Read the model definition and answer for the solid it produces. Units are mm, in the model's axes. A direction names the side the tool comes from. Give positions to 0.01 mm unless a question says otherwise; leave off trailing zeros. Write each loop counter-clockwise with the first axis right and the second up, starting at its lowest first coordinate (ties: lowest second). Pieces come first, ordered by that corner, then holes. Notation, with made-up numbers: M -19,31.25 L 7,31.25 A3 ccw 7,35.25 Z; hole C 52.5,74.5 d5. An arc over 180 degrees is marked long. Write each question's results on one line, items separated by ' | '. Start each with the question number.
```python
from build123d import *

# Parameters (mm, degrees)
F0_R          = 7.9375
F1_DEPTH      = 9.525
F1_DEPTH_BACK = 50.8
F2_R          = 31.75
F3_DEPTH      = 41.275
F4_R          = 15.08125
F5_DEPTH      = 101.601
F7_DEPTH      = 76.201


with BuildPart() as f1:
    # F0 (on Top) → F1 (new body, two sides)
    with BuildSketch(Plane.XY) as f1_sk:
        with BuildLine():
            Line((-476.25, -38.1), (0, -38.1))
            ThreePointArc((0, -38.1), (38.1, 0), (0, 38.1))
            Line((0, 38.1), (-180.615451, 38.1))
            Line((-180.615451, 38.1), (-323.73747, 38.1))
            Line((-323.73747, 38.1), (-389.728606, 0))
            Line((-389.728606, 0), (-432.606556, 0))
            ThreePointArc((-432.606556, 0), (-436.495121, 1.329884), (-438.754917, 4.7625))
            ThreePointArc((-438.754917, 4.7625), (-459.600382, 18.898166), (-476.25, 0))
            Line((-476.25, 0), (-476.25, -38.1))
        make_face()
        with Locations((-457.2, 0)):
            Circle(F0_R, mode=Mode.SUBTRACT)
    extrude(amount=F1_DEPTH)
    extrude(f1_sk.sketch, amount=-F1_DEPTH_BACK)

    # F2 (on face) → F3 (join)
    with BuildSketch(Plane.XY.offset(9.525)):
        Circle(F2_R)
    extrude(amount=F3_DEPTH)

    # F4 (on face) → F5 (cut, through all)
    with BuildSketch(Plane.XY.offset(50.8)):
        Circle(F4_R)
    extrude(amount=-F5_DEPTH, mode=Mode.SUBTRACT)

    # F6 (on face) → F7 (cut, through all)
    with BuildSketch(Plane(origin=(0, 38.1, 0), x_dir=(-1, 0, 0), z_dir=(0, 1, 0))):
        Polygon((-101.6, -50.8), (254, -50.8), (166.011819, 0), (-101.6, 0), align=None)
        Polygon((524.164035, 9.525), (168.564035, 9.525), (256.552216, -41.275), (524.164035, -41.275), align=None)
    extrude(amount=-F7_DEPTH, mode=Mode.SUBTRACT)


solid = f1.part
```
Item 1: Given P1, Ø5, axis at x = -421, z = -48, coming from the +Y side; P2, Ø1.5, axis at y = -16, z = 22.5, coming from the -X side; P3, Ø4, axis at x = -16.5, y = -19, coming from the -Z side, each flat-ended and moving along its own axis, determine where each tip first touches the part or whether it passes through.
Item 2: Section C-C, the plane x = -161 is taken. Determine the outline of the cut face in (y, z) (3 decimals).
Item 3: Section D-D, the plane z = -34 is taken. Determine the outline of the cut face in (x, y), then the cut area to 3 significant figures.
Item 4: Determine the mould class of faces 6 (the cylindrical face through (38.09, -0.84, 4.83)), 7 (the cylindrical face through (-449.868, -3.04, -45.971)), 8 (the flat face through (-411, 0, -46)), 9 (the flat face through (-210.622, 0.533, -25.756)) for opening direction Y: +Y half, -Y half, draft (parallel to the pull), parting line (faces both ways), or undercut.
Item 5: Straight lines are drawn through the part: line 1 (Y direction, x = -457.2, z = -48.5); line 2 (Y direction, x = 0, z = 38); line 3 (Z direction, x = -258, y = -17) (3 decimals). For each, find the intervals that lie inside material, in ascending order.
Item 6: For faces 1 (the flat face through (-356.3, 19.3, -46)), 2 (the flat face through (-340, -8, -41.275)), 3 (the cylindrical face through (-6.883, -30.995, 29.874)), 4 (the flat face through (14, -7, 50.8)), 5 (the flat face through (-65, 1, 0)), determine the directions among +Z, -Z, +X, -X, +Y, -Y from which every point of the face is accessible in a straight line to the end or side of a thin tool.
Item 7: Section B-B, the plane z = 25 is taken. Determine the outline of the cut face in (x, y).
Worked out:
1) P1: stops at y = 0 | P2: stops at x = -27.85 | P3: stops at z = 0
2) outline: M -38.1,0 L 38.1,0 L 38.1,9.525 L -38.1,9.525 Z
3) outline: M -243.95,-38.1 L -224.9,-38.1 L -224.9,38.1 L -243.95,38.1 Z | area: 1,450 mm²
4) face 6: parting line | face 7: undercut | face 8: +Y half | face 9: draft
5) line 1: y = -38.1 to -7.94, 7.94 to 19.05 | line 2: y = -31.75 to -15.08, 15.08 to 31.75 | line 3: z = -50.8 to -41.275
6) face 1: +Z, -Z, +Y | face 2: +Z, -X, +Y, -Y | face 3: +Z | face 4: +Z, +X, -X, +Y, -Y | face 5: -Z, +X, +Y, -Y
7) outline: C 0,0 d63.5; hole C 0,0 d30.16
